Input: part model. Units: mm. Frame: model coordinates. A direction names the side the tool comes from. Give positions to 0.01 mm unless a question says otherwise; leave off trailing zeros. Loops run counter-clockwise (first coordinate to the right, second up) from the corner with the lowest first, then second, coordinate; pieces in that order, holes last. Notation, with made-up numbers: (82, 72) -> (87, 72) arc R23 cw to (87, 111) -> close; hole circle Ø1 at (75.5, 52.5). An arc over 180 degrees is marked (long way). Answer in a Markdown table with one row per item. Add a question column.
```python
from build123d import *

# Parameters (mm, degrees)
F0_R     = 1.2295
F0_R_2   = 1.5
F1_DEPTH = 6


# Not quite as in the source:
# - ends of sketch curves that miss each other by under 0.0002 mm in the source are joined


with BuildPart() as f1:
    # F0 (on Top) → F1 (new body)
    with BuildSketch(Plane.XY):
        Polygon((-110, -103), (-110, -107), (-107, -110), (-103, -110), (-83, -90), (-63, -90), (-53, -100), (-15, -100), (-5, -90), (5, -90), (15, -100), (53, -100), (63, -90), (83, -90), (103, -110), (107, -110), (110, -107), (110, -103), (85, -78), (85, 78), (110, 103), (110, 107), (107, 110), (103, 110), (63, 70), (43, 70), (13, 100), (-13, 100), (-43, 70), (-63, 70), (-103, 110), (-107, 110), (-110, 107), (-110, 103), (-85, 78), (-85, -78), align=None)
        with Locations((-104.5, -104.5)):
            Circle(F0_R, mode=Mode.SUBTRACT)
        with Locations((-34.999989, -95.000012)):
            Circle(F0_R_2, mode=Mode.SUBTRACT)
        with BuildLine():
            ThreePointArc((-20.007037, -86), (-21.1786098753, -88.8284271247), (-24.007037, -90))
            Line((-24.007037, -90), (-47.007037, -90))
            ThreePointArc((-47.007037, -90), (-49.8354641247, -88.8284271247), (-51.007037, -86))
            Line((-51.007037, -86), (-51.007037, -84))
            ThreePointArc((-51.007037, -84), (-49.8354641247, -81.1715728753), (-47.007037, -80))
            Line((-47.007037, -80), (-24.007037, -80))
            ThreePointArc((-24.007037, -80), (-21.1786098753, -81.1715728753), (-20.007037, -84))
            Line((-20.007037, -84), (-20.007037, -86))
        make_face(mode=Mode.SUBTRACT)
        with Locations((-34.999989, -75.000012)):
            Circle(F0_R_2, mode=Mode.SUBTRACT)
        with Locations((35.000011, -95.000012)):
            Circle(F0_R_2, mode=Mode.SUBTRACT)
        with BuildLine():
            ThreePointArc((50, -86), (48.8284271247, -88.8284271247), (46, -90))
            Line((46, -90), (23, -90))
            ThreePointArc((23, -90), (20.1715728753, -88.8284271247), (19, -86))
            Line((19, -86), (19, -84))
            ThreePointArc((19, -84), (20.1715728753, -81.1715728753), (23, -80))
            Line((23, -80), (46, -80))
            ThreePointArc((46, -80), (48.8284271247, -81.1715728753), (50, -84))
            Line((50, -84), (50, -86))
        make_face(mode=Mode.SUBTRACT)
        with Locations((35.000011, -75.000012)):
            Circle(F0_R_2, mode=Mode.SUBTRACT)
        with Locations((104.5, -104.5)):
            Circle(F0_R, mode=Mode.SUBTRACT)
        Polygon((25, -60), (5, -80), (-5, -80), (-25, -60), (-25, -40), (-5, -20), (5, -20), (25, -40), align=None, mode=Mode.SUBTRACT)
        Polygon((-75, -68), (-75, 68), (-35, 28), (-35, -28), align=None, mode=Mode.SUBTRACT)
        with Locations((-20, 0)):
            Circle(F0_R, mode=Mode.SUBTRACT)
        with Locations((-104.5, 104.5)):
            Circle(F0_R, mode=Mode.SUBTRACT)
        with BuildLine():
            Line((-16.5, -8.2), (-16.5, 8.2))
            Line((-16.5, 8.2), (-11.5, 8.2))
            Line((-11.5, 8.2), (-11.5, 2.5))
            ThreePointArc((-11.5, 2.5), (-11.2071067812, 1.7928932188), (-10.5, 1.5))
            Line((-10.5, 1.5), (-2.662278, 1.5))
            ThreePointArc((-2.662278, 1.5), (0.4999997857, 3.5), (3.6622775389, 1.5000002556))
            Line((3.6622775389, 1.5000002556), (11.5, 1.5))
            ThreePointArc((11.5, 1.5), (12.2071067812, 1.7928932188), (12.5, 2.5))
            Line((12.5, 2.5), (12.5, 8.2))
            Line((12.5, 8.2), (17.5, 8.2))
            Line((17.5, 8.2), (17.5, -8.2))
            Line((17.5, -8.2), (12.5, -8.2))
            Line((12.5, -8.2), (12.5, -2.5))
            ThreePointArc((12.5, -2.5), (12.2071067812, -1.7928932188), (11.5, -1.5))
            Line((11.5, -1.5), (3.662277, -1.5))
            ThreePointArc((3.662277, -1.5), (0.4999997857, -3.5), (-2.6622777226, -1.4999998684))
            Line((-2.6622777226, -1.4999998684), (-10.5, -1.5))
            ThreePointArc((-10.5, -1.5), (-11.2071067812, -1.7928932188), (-11.5, -2.5))
            Line((-11.5, -2.5), (-11.5, -8.2))
            Line((-11.5, -8.2), (-16.5, -8.2))
        make_face(mode=Mode.SUBTRACT)
        with Locations((21, 0)):
            Circle(F0_R, mode=Mode.SUBTRACT)
        Polygon((-5, 20), (-25, 40), (-25, 50), (-5, 70), (5, 70), (25, 50), (25, 40), (5, 20), align=None, mode=Mode.SUBTRACT)
        Polygon((75, 68), (75, -68), (35, -28), (35, 28), align=None, mode=Mode.SUBTRACT)
        with Locations((1.1e-05, 74.999988)):
            Circle(F0_R_2, mode=Mode.SUBTRACT)
        with BuildLine():
            ThreePointArc((16.137123, 84), (14.9655501247, 81.1715728753), (12.137123, 80))
            Line((12.137123, 80), (-10.862877, 80))
            ThreePointArc((-10.862877, 80), (-13.6913041247, 81.1715728753), (-14.862877, 84))
            Line((-14.862877, 84), (-14.862877, 86))
            ThreePointArc((-14.862877, 86), (-13.6913041247, 88.8284271247), (-10.862877, 90))
            Line((-10.862877, 90), (12.137123, 90))
            ThreePointArc((12.137123, 90), (14.9655501247, 88.8284271247), (16.137123, 86))
            Line((16.137123, 86), (16.137123, 84))
        make_face(mode=Mode.SUBTRACT)
        with Locations((1.1e-05, 94.999988)):
            Circle(F0_R_2, mode=Mode.SUBTRACT)
        with Locations((104.5, 104.5)):
            Circle(F0_R, mode=Mode.SUBTRACT)
    extrude(amount=F1_DEPTH)


solid = f1.part
```
1) Section D-D on x = -78.5. Output: boundary loops of the cut face in (y, z).
2) Section A-A on y = -45. Output: boundary loops of the cut face in (x, z).
3) Material intervals for line 1 along Y through (x, z) = (43.5, 1.3); line 2 along Y through (x, z) = (38.5, 4.4); line 3 along X through (y, z) = (16.5, 4.7), sorted ascending.
4) Pull-direction query (X, two-part tool) for faces 5 (the face through (-7, 1.5, 3)), 6 (the face through (-98, 91, 3)), 7 (the face through (-26, 2, 6)); classes: +X half, -X half, draft (parallel to the pull), parting line (faces both ways), or undercut.
5) Pin query (flat end, axial travel): pin 1 (0.6 mm diameter, centred on y = 85.5, z = 4.5, fed in from +X); pin 2 (3 mm diameter, centred on x = 78, z = 3.5, fed in from -Y); pin 3 (1.8 mm diameter, centred on x = 51, z = 1.5, fed in from +Y). Return the tip coordinate at first contact, or that it passes through.
6) Section C-C on z = 4.3. State how many separate pieces and enclosed holes the cut face has, and give its area (3 significant figures).
7) Reachability of faces 1 (the face through (-85, 1, 3)), 2 (the face through (-15, 60, 3)), 3 (the face through (85, -1, 3)), 4 (the face through (73, -90, 3)) from +Z, -Z, +X, -X, +Y, -Y: full face, straight path, thin tool, end or side. Return the list, or none.
8) Section B-B on x = 57.5. Output: boundary loops of the cut face in (y, z), and give its area (3 significant figures).
Working result:
| question | item | result |
|---|---|---|
| 1 | outline | (-90, 0) -> (85.5, 0) -> (85.5, 6) -> (-90, 6) -> close |
| 2 | outline | (-85, 0) -> (-75, 0) -> (-75, 6) -> (-85, 6) -> close; (-52, 0) -> (-25, 0) -> (-25, 6) -> (-52, 6) -> close; (25, 0) -> (52, 0) -> (52, 6) -> (25, 6) -> close; (75, 0) -> (85, 0) -> (85, 6) -> (75, 6) -> close |
| 3 | line 1 | y = -100 to -90, -80 to -36.5, 36.5 to 70 |
| 3 | line 2 | y = -100 to -90, -80 to -31.5, 31.5 to 74.5 |
| 3 | line 3 | x = -85 to -75, -35 to 35, 75 to 85 |
| 4 | face 5 | undercut |
| 4 | face 6 | -X half |
| 4 | face 7 | draft |
| 5 | pin 1 | stops at x = 92.8 |
| 5 | pin 2 | stops at y = -90 |
| 5 | pin 3 | stops at y = 70 |
| 6 | separate pieces | 1 |
| 6 | enclosed holes | 20 |
| 6 | area | 18,800 mm2 |
| 7 | face 1 | +Z, -Z, -X |
| 7 | face 2 | +Z, -Z |
| 7 | face 3 | +Z, -Z, +X |
| 7 | face 4 | +Z, -Z, -Y |
| 8 | outline | (-95.5, 0) -> (-50.5, 0) -> (-50.5, 6) -> (-95.5, 6) -> close; (50.5, 0) -> (70, 0) -> (70, 6) -> (50.5, 6) -> close |
| 8 | area | 387 mm2 |
